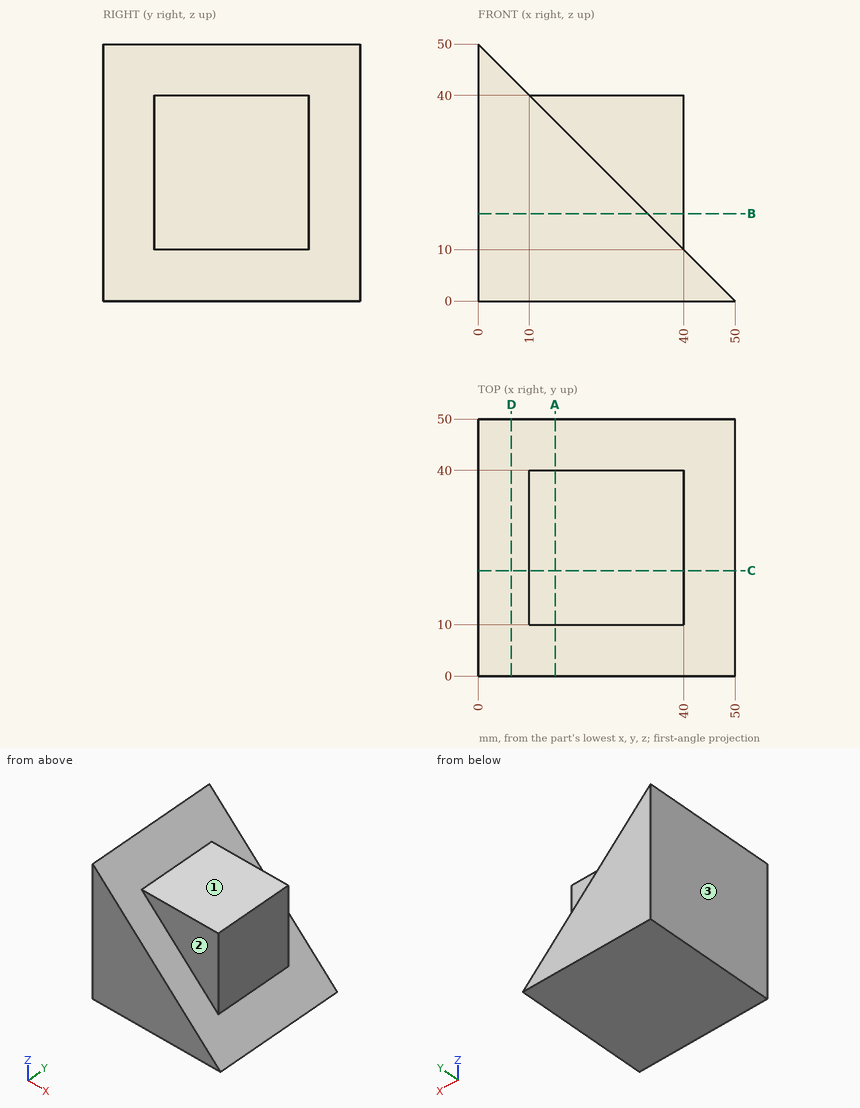
Geometry check sheet. Reference: drawing and pictorial views, mm from the part's lowest x, y, z. A direction names the side the tool comes from. Give positions to 0.01 mm unless a question says otherwise; leave off trailing zeros. Order: outer loops, then holes, each group sorted by start corner. A loop starts at its lowest first (then second) coordinate and runs counter-clockwise, first axis right, second up. Notation, with made-up numbers: M 51,-22 L 60,-22 A16 ccw 60,-8 Z; hole C -38,58.5 d9. An arc over 180 degrees is marked long. Answer as CSV lines item,"result". Start each with the question number.
Item 1: Tool access check on the marked faces 1, 2 and 3. Record the directions out of +Z, -Z, +X, -X, +Y, -Y that give a thin tool (end or side, any length) a straight path to the whole face; none if there is none.
Item 2: Thickness scan on line 1 (X direction, y = 19.5, z = 29.5); line 2 (Y direction, x = 35.5, z = 30.5). Record the ranges inside material, lowest first. Write a range as [from, to].
Item 3: Cross-section at A-A on x = 15. Enter the section's corners in (y, z), plus the area to 3 significant figures.
Item 4: Gauge pin test, flat ends, axial feed: P1, Ø1, axis at x = 32, y = 29, coming from the +Z side; P2, Ø9, axis at y = 30.5, z = 20.5, coming from the +X side; P3, Ø6, axis at x = 20.5, z = 40, coming from the -Y side. Record the tip position at first contact, or that the pin passes through.
Item 5: Cross-section at B-B on z = 17. Enter the section's corners in (x, y).
Item 6: Cross-section at D-D on x = 6.5. Enter the section's corners in (y, z), plus the area to 4 significant figures.
Item 7: Cross-section at C-C on y = 20.5. Enter the section's corners in (x, z).
Established:
1,face 1,"+Z, +X, +Y, -Y"
1,face 2,"+Z, +X, -Y"
1,face 3,"+Z, -Z, -X, +Y, -Y"
2,line 1,"x = [0, 40]"
2,line 2,"y = [10, 40]"
3,outline,"M 0,0 L 50,0 L 50,35 L 40,35 L 40,40 L 10,40 L 10,35 L 0,35 Z"
3,area,"1,900 mm^2"
4,P1,"stops at z = 40"
4,P2,"stops at x = 40"
4,P3,"stops at y = 10"
5,outline,"M 0,0 L 33,0 L 33,10 L 40,10 L 40,40 L 33,40 L 33,50 L 0,50 Z"
6,outline,"M 0,0 L 50,0 L 50,43.5 L 0,43.5 Z"
6,area,"2,175 mm^2"
7,outline,"M 0,0 L 50,0 L 40,10 L 40,40 L 10,40 L 0,50 Z"
